```python
from build123d import *

# Parameters (mm, degrees)
SKETCH1_R               = 2.05
BOSS_EXTRUDE1_DEPTH     = 5
SKETCH2_W               = 1
SKETCH2_H               = 5
CUT_EXTRUDE_THIN1_DEPTH = 2


with BuildPart() as part:
    # Sketch1 → Boss-Extrude1 (new body)
    with BuildSketch(Plane.XY):
        with BuildLine():
            Line((0, 3.25), (18, 3.25))
            ThreePointArc((18, 3.25), (21.25, 0), (18, -3.25))
            Line((18, -3.25), (0, -3.25))
            ThreePointArc((0, -3.25), (-3.25, 0), (0, 3.25))
        make_face()
        Circle(SKETCH1_R, mode=Mode.SUBTRACT)
        with Locations((18, 0)):
            Circle(SKETCH1_R, mode=Mode.SUBTRACT)
        with BuildLine():
            Line((11.5, -2), (6.5, -2))
            ThreePointArc((6.5, -2), (4.5, 0), (6.5, 2))
            Line((6.5, 2), (11.5, 2))
            ThreePointArc((11.5, 2), (13.5, 0), (11.5, -2))
        make_face(mode=Mode.SUBTRACT)
    extrude(amount=BOSS_EXTRUDE1_DEPTH)

    # Sketch2 → Cut-Extrude-Thin1 (cut)
    with BuildSketch(Plane(origin=(0, -3.25, 0), x_dir=(-1, 0, 0), z_dir=(0, -1, 0))):
        with Locations((0, -2.5)):
            Rectangle(SKETCH2_W, SKETCH2_H)
        with Locations((-18, -2.5)):
            Rectangle(SKETCH2_W, SKETCH2_H)
    extrude(amount=-CUT_EXTRUDE_THIN1_DEPTH, mode=Mode.SUBTRACT)


solid = part.part
```
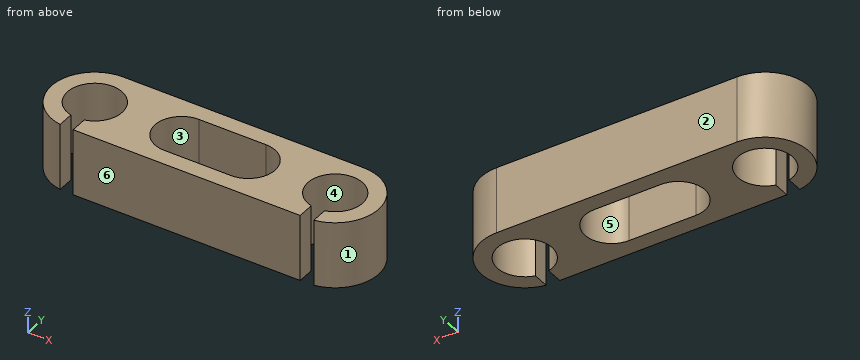
Design review of the part built by this model. Coordinates are the model's own, in mm. Face numbers are marked on the shaded views. A direction names the side the tool comes from. Coordinates: 2 decimals unless noted, no trailing zeros. Loops run counter-clockwise (first coordinate to the right, second up) from the corner with the lowest first, then second, coordinate; pieces in that order, holes last. Notation, with made-up numbers: M 68.25,71.5 L 123.25,71.5 A32 cw 123.25,98.5 Z; hole C -27.5,-7.5 d10. An arc over 180 degrees is marked long. One line per question, with ' | ' between items.
(1) Wall thickness on probe 1 along X at (y, z) = (0, 1.75); probe 2 along X at (y, z) = (-1.25, 0.95); probe 3 along X at (y, z) = (-2.5, 3.95): over which ranges is each line inside the solid? List them lowest first.
Filled in:
probe 1: x = -3.25 to -2.05, 2.05 to 4.5, 13.5 to 15.95, 20.05 to 21.25 | probe 2: x = -3 to -1.62, 1.62 to 4.94, 13.06 to 16.38, 19.62 to 21 | probe 3: x = -2.08 to -0.5, 0.5 to 17.5, 18.5 to 20.08
(2) We need section B-B (y = 0). Give the boundary of the cut face in (x, z).
Filled in:
outline: M -3.25,0 L -2.05,0 L -2.05,5 L -3.25,5 Z; M 2.05,0 L 4.5,0 L 4.5,5 L 2.05,5 Z; M 13.5,0 L 15.95,0 L 15.95,5 L 13.5,5 Z; M 20.05,0 L 21.25,0 L 21.25,5 L 20.05,5 Z
(3) We need section C-C (y = -1). Give the boundary of the cut face in (x, z).
Filled in:
outline: M -3.09,0 L -1.79,0 L -1.79,5 L -3.09,5 Z; M 1.79,0 L 4.77,0 L 4.77,5 L 1.79,5 Z; M 13.23,0 L 16.21,0 L 16.21,5 L 13.23,5 Z; M 19.79,0 L 21.09,0 L 21.09,5 L 19.79,5 Z
(4) We need section A-A (z = 1.35). Give the boundary of the cut face in (x, y), and give its area (3 significant figures).
Filled in:
outline: M -0.5,-3.21 L -0.5,-1.99 A2.05 cw long 0.5,-1.99 L 0.5,-3.25 L 17.5,-3.25 L 17.5,-1.99 A2.05 cw long 18.5,-1.99 L 18.5,-3.21 A3.25 ccw 18,3.25 L 0,3.25 A3.25 ccw Z; hole M 6.5,-2 L 11.5,-2 A2 ccw 11.5,2 L 6.5,2 A2 ccw Z | area: 88.8 mm^2
(5) Draft analysis for pull direction X (two halves, no side actions). For the marked faces 1, 2, 3 and 4, state which applies: released by +X, released by -X, zero draft, split by the parting line, or undercut.
Filled in:
face 1: released by +X | face 2: zero draft | face 3: undercut | face 4: undercut
(6) For pin 1 Ø1.3 at (y, z) = (-2.5, 2.5) entering from +X; pin 2 Ø1 at (y, z) = (-2.5, 2.5) entering from +X; pin 3 Ø1 at (y, z) = (-2.5, 3) entering from -X, all flat-tipped, find the tip position at first contact; note any pin that passes through.
Filled in:
pin 1: stops at x = 20.67 | pin 2: stops at x = 20.56 | pin 3: stops at x = -2.56
(7) Machinability: for the marked faces 5 and 6, which of the approach directions +Z, -Z, +X, -X, +Y, -Y give a long, thin tool a straight path to every point of the face, cutting with its end or side? Answer none if there is none.
Filled in:
face 5: +Z, -Z | face 6: +Z, -Z, +X, -X, -Y
